Work out the finished part from the listing and answer in its coordinate system (mm). A direction names the side the tool comes from. Give positions to 0.01 mm unless a question says otherwise; leave off trailing zeros. Write each loop counter-clockwise with the first axis right and the second up, starting at its lowest first coordinate (ties: lowest second). Pieces come first, ordered by that corner, then holes. Notation, with made-up numbers: (-29.75, 46.5) -> (26.25, 46.5) arc R32 cw to (26.25, 77.5) -> close; hole circle Ø9 at (-29.75, -6.5). An arc over 180 degrees is marked (long way). Use a Markdown table: item, result. Add a question column.
Q1. Section A-A, the plane z = 2.05 is taken. State how many separate pieces and enclosed holes the cut face has, plus the area to 3 significant figures.
Q2. Consider line 1 (X direction, y = -48, z = 1.6); line 2 (X direction, y = 10.5, z = 0.95); line 3 (Y direction, x = 30.5, z = 2.15). Determine where each line is inside the solid, lowest interval first.
Q3. Each of these flat-tipped pins is pushed along its axis until it touches: pin 1 Ø0.9 at (y, z) = (-49.5, 1.5) entering from -X; pin 2 Ø10 at (x, y) = (-11, -33.5) entering from -Z; pin 3 Ø0.9 at (y, z) = (-51, 1) entering from +X; pin 4 Ø1.5 at (y, z) = (-24, 1) entering from +X. Where does it stop, or does it pass through?
Q4. For faces 1 (the face through (40, -25, 1)), 2 (the face through (30, -45, 1)), 3 (the face through (-40, 25, 1)), 4 (the face through (0, -60, 1)), 5 (the face through (48, 24, 1)), determine the directions among +Z, -Z, +X, -X, +Y, -Y from which every point of the face is accessible in a straight line to the end or side of a thin tool.
Q5. For a pull along Y with two mould halves and no side action, classify faces 6 (the face through (32.5, -50, 1)), 7 (the face through (-35, 40, 1)), 8 (the face through (-33, -59, 1)) as pulls with the +Y half, pulls with the -Y half, needs draft (parallel to the pull), parting line crosses it, or undercut.
Q6. Section B-B, the plane y = 35 is taken. Give the vertices of the cut face in (x, z), plus the area to 3 significant figures.
Autodesk Fusion 360 part; units mm, degrees
sketch "Sketch1" plane through (0, 0, 0) normal (0, 0, 1) x (1, 0, 0)
  line L0 (30, 50) -> (-30, 50)
  line L1 (-30, 50) -> (-30, -50)
  line L2 (-30, -50) -> (30, -50)
  line L3 (30, -50) -> (30, 50)
  line L4 (30, 50) -> (-30, -50) construction
  line L5 (-30, 50) -> (30, -50) construction
  line L6 (45, 25) -> (-45, 25)
  line L7 (-50, 20) -> (-50, -20)
  line L8 (-45, -25) -> (45, -25)
  line L9 (50, -20) -> (50, 20)
  line L10 (50, 25) -> (-50, -25) construction
  line L11 (-50, 25) -> (50, -25) construction
  line L12 (35, 10.5) -> (-35, 10.5) construction
  line L13 (-35, 10.5) -> (-35, -10.5) construction
  line L14 (-35, -10.5) -> (35, -10.5) construction
  line L15 (35, -10.5) -> (35, 10.5) construction
  line L16 (35, 10.5) -> (-35, -10.5) construction
  line L17 (-35, 10.5) -> (35, -10.5) construction
  circle A0 centre (-35, 10.5) radius 3
  circle A1 centre (-35, -10.5) radius 3
  circle A2 centre (35, 10.5) radius 3
  circle A3 centre (35, -10.5) radius 3
  line L18 (-27.5, 47.5) -> (-27.5, 52.5)
  arc A4 (-27.5, 52.5) -> (-32.5, 52.5) centre (-30, 52.5) ccw
  line L19 (-32.5, 52.5) -> (-32.5, 47.5)
  arc A5 (-32.5, 47.5) -> (-27.5, 47.5) centre (-30, 47.5) ccw
  line L20 (-30, 47.5) -> (-30, 52.5) construction
  line L21 (32.5, 47.5) -> (32.5, 52.5)
  arc A6 (32.5, 52.5) -> (27.5, 52.5) centre (30, 52.5) ccw
  line L22 (27.5, 52.5) -> (27.5, 47.5)
  arc A7 (27.5, 47.5) -> (32.5, 47.5) centre (30, 47.5) ccw
  line L23 (30, 47.5) -> (30, 52.5) construction
  line L24 (-70, 0) -> (55, 0) construction
  arc A8 (-32.5, -52.5) -> (-27.5, -52.5) centre (-30, -52.5) ccw
  line L25 (-32.5, -52.5) -> (-32.5, -47.5)
  line L26 (-27.5, -47.5) -> (-27.5, -52.5)
  arc A9 (-27.5, -47.5) -> (-32.5, -47.5) centre (-30, -47.5) ccw
  arc A10 (32.5, -47.5) -> (27.5, -47.5) centre (30, -47.5) ccw
  arc A11 (27.5, -52.5) -> (32.5, -52.5) centre (30, -52.5) ccw
  line L27 (27.5, -52.5) -> (27.5, -47.5)
  line L28 (32.5, -47.5) -> (32.5, -52.5)
  line L29 (30, 60) -> (-30, 60)
  line L30 (-35, 55) -> (-35, -55)
  line L31 (-30, -60) -> (30, -60)
  line L32 (35, -55) -> (35, 55)
  line L33 (35, 60) -> (-35, -60) construction
  line L34 (-35, 60) -> (35, -60) construction
  arc A12 (-30, 60) -> (-35, 55) centre (-30, 55) ccw
  arc A13 (35, 55) -> (30, 60) centre (30, 55) ccw
  arc A14 (-35, -55) -> (-30, -60) centre (-30, -55) ccw
  arc A15 (30, -60) -> (35, -55) centre (30, -55) ccw
  arc A16 (-27.5, -50.0014) -> (-27.5, -49.9986) centre (-30, -50) ccw
  arc A17 (-32.5, -49.9986) -> (-32.5, -50.0014) centre (-30, -50) ccw
  arc A18 (-32.5, 50.0024) -> (-32.5, 49.9976) centre (-30, 50) ccw
  arc A19 (-27.5, 50) -> (-27.5, 50.0014) centre (-30, 50) ccw
  arc A20 (50, 20) -> (45, 25) centre (45, 20) ccw
  arc A21 (45, -25) -> (50, -20) centre (45, -20) ccw
  arc A22 (-50, -20) -> (-45, -25) centre (-45, -20) ccw
  arc A23 (-45, 25) -> (-50, 20) centre (-45, 20) ccw
  point P0 (-30, 50)
  point P1 (30, 50)
  dimension "d1" = 60
  dimension "d2" = 100
  dimension "d5" = 5
  dimension "d7" = 100
  dimension "d8" = 50
  dimension "d9" = 70
  dimension "d10" = 21
  dimension "d12" = 6
  dimension "d13" = 6
  dimension "d14" = 6
  dimension "d15" = 6
  dimension "d16" = 5
  dimension "d17" = 70
  dimension "d18" = 120
  dimension "d19" = 5
  dimension "d20" = 5
extrude "Extrude1" add sketch "Sketch1" along normal blind 3 contours L0 L1 L3 L6 L18 A4 L19 A5 L21 A6 L22 A7 L29 L30 L32 A12 A13 A18 A19 | L0 L1 L3 L6 L18 A5 L22 A7 | L1 L3 L6 L8 | L1 L6 L8 A0 A1 L30 | L3 L6 L8 A2 A3 L32 | L1 L2 L3 L8 L26 A9 A10 L27 | L1 L2 L3 L8 A8 L25 L26 A9 A10 A11 L27 L28 L30 L31 L32 A14 A15 A17 | L6 L7 L8 A0 A1 L30 A22 A23 | L6 L8 L9 A2 A3 L32 A20 A21
sketch "dfx_export" plane through (0, 0, 3) normal (0, 0, 1) x (1, 0, 0)
  arc A0 (-27.5, -47.5) -> (-32.5, -47.5) centre (-30, -47.5) ccw
  line L0 (-27.5, -47.5) -> (-27.5, -49.9986)
  arc A1 (-27.5, -50.0014) -> (-27.5, -49.9986) centre (-30, -50) ccw
  line L1 (-27.5, -50.0014) -> (-27.5, -52.5)
  arc A2 (-32.5, -52.5) -> (-27.5, -52.5) centre (-30, -52.5) ccw
  line L2 (-32.5, -52.5) -> (-32.5, -50.0014)
  arc A3 (-32.5, -49.9986) -> (-32.5, -50.0014) centre (-30, -50) ccw
  line L3 (-32.5, -49.9986) -> (-32.5, -47.5)
  arc A4 (27.5, 47.5) -> (32.5, 47.5) centre (30, 47.5) ccw
  line L4 (27.5, 47.5) -> (27.5, 52.5)
  arc A5 (32.5, 52.5) -> (27.5, 52.5) centre (30, 52.5) ccw
  line L5 (32.5, 52.5) -> (32.5, 47.5)
  arc A6 (-27.5, 50) -> (-27.5, 50.0014) centre (-30, 50) ccw
  line L6 (-27.5, 50) -> (-27.5, 47.5)
  arc A7 (-32.5, 47.5) -> (-27.5, 47.5) centre (-30, 47.5) ccw
  line L7 (-32.5, 47.5) -> (-32.5, 49.9976)
  arc A8 (-32.5, 50.0024) -> (-32.5, 49.9976) centre (-30, 50) ccw
  line L8 (-32.5, 50.0024) -> (-32.5, 52.5)
  arc A9 (-27.5, 52.5) -> (-32.5, 52.5) centre (-30, 52.5) ccw
  line L9 (-27.5, 52.5) -> (-27.5, 50.0014)
  arc A10 (27.5, -52.5) -> (32.5, -52.5) centre (30, -52.5) ccw
  line L10 (27.5, -52.5) -> (27.5, -47.5)
  arc A11 (32.5, -47.5) -> (27.5, -47.5) centre (30, -47.5) ccw
  line L11 (32.5, -47.5) -> (32.5, -52.5)
  circle A12 centre (35, -10.5) radius 3
  circle A13 centre (35, 10.5) radius 3
  circle A14 centre (-35, 10.5) radius 3
  circle A15 centre (-35, -10.5) radius 3
  arc A16 (-45, 25) -> (-50, 20) centre (-45, 20) ccw
  line L12 (-50, 20) -> (-50, -20)
  arc A17 (-50, -20) -> (-45, -25) centre (-45, -20) ccw
  line L13 (-45, -25) -> (-35, -25)
  line L14 (-35, -25) -> (-35, -55)
  arc A18 (-35, -55) -> (-30, -60) centre (-30, -55) ccw
  line L15 (-30, -60) -> (30, -60)
  arc A19 (30, -60) -> (35, -55) centre (30, -55) ccw
  line L16 (35, -55) -> (35, -25)
  line L17 (35, -25) -> (45, -25)
  arc A20 (45, -25) -> (50, -20) centre (45, -20) ccw
  line L18 (50, -20) -> (50, 20)
  arc A21 (50, 20) -> (45, 25) centre (45, 20) ccw
  line L19 (45, 25) -> (35, 25)
  line L20 (35, 25) -> (35, 55)
  arc A22 (35, 55) -> (30, 60) centre (30, 55) ccw
  line L21 (30, 60) -> (-30, 60)
  arc A23 (-30, 60) -> (-35, 55) centre (-30, 55) ccw
  line L22 (-35, 55) -> (-35, 25)
  line L23 (-35, 25) -> (-45, 25)
Result set:
| question | item | result |
|---|---|---|
| 1 | separate pieces | 1 |
| 1 | enclosed holes | 8 |
| 1 | area | 9,570 mm2 |
| 2 | line 1 | x = -35 to -32.5, -27.5 to 27.5, 32.5 to 35 |
| 2 | line 2 | x = -50 to -38, -32 to 32, 38 to 50 |
| 2 | line 3 | y = -59.97 to -54.95, -45.05 to 45.05, 54.95 to 59.97 |
| 3 | pin 1 | stops at x = -35 |
| 3 | pin 2 | stops at z = 0 |
| 3 | pin 3 | stops at x = 35 |
| 3 | pin 4 | stops at x = 48.8 |
| 4 | face 1 | +Z, -Z, +X, -Y |
| 4 | face 2 | +Z, -Z |
| 4 | face 3 | +Z, -Z, -X, +Y |
| 4 | face 4 | +Z, -Z, +X, -X, -Y |
| 4 | face 5 | +Z, -Z, +X, +Y |
| 5 | face 6 | undercut |
| 5 | face 7 | needs draft |
| 5 | face 8 | pulls with the -Y half |
| 6 | outline | (-35, 0) -> (35, 0) -> (35, 3) -> (-35, 3) -> close |
| 6 | area | 210 mm2 |
